For this review, take the finished solid that the model builds, in its own axes (mm). Face numbers are marked on the shaded views. A direction names the side the tool comes from. Coordinates: 2 decimals unless noted, no trailing zeros. Order: outer loops, then holes, each group sorted by start corner. A loop starts at its lowest first (then second) coordinate and runs counter-clockwise, first axis right, second up. Notation, with made-up numbers: (38.5, 33.5) - (76.5, 33.5) arc R16 ccw to (76.5, 63.5) - close; hole circle Ø7 at (84, 89). An arc over 180 degrees is marked (long way). One line per item, written item: value. Start each with the question number.
(1) Consider section A-A on x = 56.75. Write out the cut boundary in (y, z), then the cut area to 3 significant figures.
(2) Mouldability with a two-part tool opening along X and no side actions: class the marked faces 4, 5 and 6 as released by +X, released by -X, zero draft, split by the parting line, or undercut.
(3) For the marked faces 1, 2 and 3, list the 3-axis set-ups (+Z, -Z, +X, -X, +Y, -Y) from which the entire face can be reached by the end or side of a thin tool; tool diameter is ignored.
(4) Consider section D-D on z = 17.5. Write out the cut boundary in (x, y), then the cut area to 3 significant figures.
(5) To check wall thickness, follow line 1 along X through (y, z) = (13.5, 16.75); line 2 along X through (y, z) = (1.5, 18.25); line 3 along Y through (x, z) = (27.5, 9.5). State the ranges of each line that lie inside material, in increasing order.
(6) Consider section B-B on y = 4.25. Write out the cut boundary in (x, z).
(7) Clearance check with flat-ended pins moving along their axes: pin 1 (7 mm diameter, centred on x = 57, z = 10.5, fed in from +Y); pin 2 (6.5 mm diameter, centred on x = -54.5, z = 10, fed in from +Y); pin 3 (2 mm diameter, centred on x = 56.75, z = 10, fed in from +Y); pin 4 (5 mm diameter, centred on y = 15, z = 11, fed in from -X). State where each tip first meets the part, or that it passes through.
(8) Consider section C-C on y = 16.75. Write out the cut boundary in (x, z).
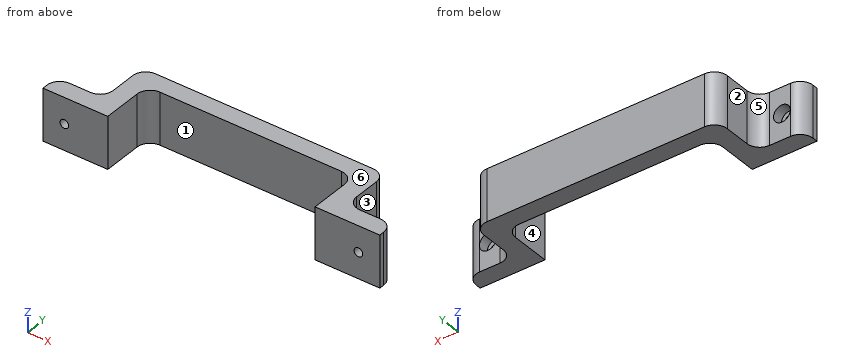
```python
from build123d import *

# Parameters (mm, degrees)
F1_DEPTH = 20
F2_R     = 5
F4_R     = 3.25
F5_DEPTH = 25
F6_R     = 1.65
F7_DEPTH = 25


with BuildPart() as f1:
    # F0 (on Top) → F1 (new body)
    with BuildSketch(Plane.XY):
        Polygon((-40, 20), (0, 20), (40, 20), (40, 0), (65, 0), (65, 7), (47, 7), (47, 27), (0, 27), (-47, 27), (-47, 7), (-65, 7), (-65, 0), (-40, 0), align=None)
    extrude(amount=F1_DEPTH)

    # F2
    f2_edges = [f1.edges().sort_by_distance(p)[0] for p in [
        (40, 20, 10),
        (47, 27, 10),
        (-40, 20, 10),
        (-47, 27, 10),
        (47, 7, 10),
        (-47, 7, 10),
        (65, 7, 10),
        (-65, 7, 10),
    ]]
    fillet(f2_edges, radius=F2_R)

    # F4 (on offset) → F5 (cut)
    with BuildSketch(Plane.XZ.offset(-3)):
        with Locations((-56.75, 10)):
            Circle(F4_R)
        with Locations((56.75, 10)):
            Circle(F4_R)
    extrude(amount=-F5_DEPTH, mode=Mode.SUBTRACT)

    # F6 (on face) → F7 (cut)
    with BuildSketch(Plane(origin=(0, 3, 0), x_dir=(-1, 0, 0), z_dir=(0, 1, 0))):
        with Locations((-56.75, 10)):
            Circle(F6_R)
        with Locations((56.75, 10)):
            Circle(F6_R)
    extrude(amount=-F7_DEPTH, mode=Mode.SUBTRACT)


solid = f1.part
```
Geometry check:
1. outline: (0, 0) - (7, 0) - (7, 6.75) - (3, 6.75) - (3, 8.35) - (0, 8.35) - close; (0, 11.65) - (3, 11.65) - (3, 13.25) - (7, 13.25) - (7, 20) - (0, 20) - close
1. area: 104 mm^2
2. face 4: undercut
2. face 5: released by -X
2. face 6: zero draft
3. face 1: +Z, -Z, -Y
3. face 2: +Z, -Z, -X, +Y
3. face 3: +Z, -Z, +X, +Y
4. outline: (-65, 0) - (-40, 0) - (-40, 15) arc R5 cw to (-35, 20) - (35, 20) arc R5 cw to (40, 15) - (40, 0) - (65, 0) - (65, 2) arc R5 ccw to (60, 7) - (52, 7) arc R5 cw to (47, 12) - (47, 22) arc R5 ccw to (42, 27) - (-42, 27) arc R5 ccw to (-47, 22) - (-47, 12) arc R5 cw to (-52, 7) - (-60, 7) arc R5 ccw to (-65, 2) - close
4. area: 1,190 mm^2
5. line 1: x = -47 to -40, 40 to 47
5. line 2: x = -65 to -40, 40 to 65
5. line 3: y = 20 to 27
6. outline: (-64.47, 0) - (-40, 0) - (-40, 20) - (-64.47, 20) - close; (40, 0) - (64.47, 0) - (64.47, 20) - (40, 20) - close; hole circle Ø6.5 at (-56.75, 10); hole circle Ø6.5 at (56.75, 10)
7. pin 1: stops at y = 7
7. pin 2: stops at y = 7.06
7. pin 3: passes through
7. pin 4: stops at x = -47
8. outline: (-47, 0) - (-39.68, 0) - (-39.68, 20) - (-47, 20) - close; (39.68, 0) - (47, 0) - (47, 20) - (39.68, 20) - close
